Design review of the part built by this model. Coordinates are the model's own, in mm. A direction names the side the tool comes from. Coordinates: 2 decimals unless noted, no trailing zeros. Write each loop counter-clockwise with the first axis right and the second up, starting at its lowest first coordinate (ties: lowest second). Pieces come first, ordered by that corner, then holes. Notation, with made-up numbers: (12, -17.75) -> (31, -17.75) arc R26 cw to (31, 19.25) -> close; hole circle Ø2 at (-20.5, 26.5). An arc over 180 degrees is marked (long way). Answer in a Markdown table with one row per item. Add a question column.
Item 1: Take a section at A-A, the plane x = 0. Give the number of separate pieces and of enclosed holes in the cut face, and give its area (3 significant figures).
Item 2: To check wall thickness, follow line 1 (Z direction, x = -0.05, y = 2.05); line 2 (X direction, y = 3.2, z = 0) (3 decimals); line 3 (Z direction, x = -0.1, y = 0.2). State the ranges of each line that lie inside material, in increasing order.
Item 3: Take a section at B-B, the plane z = 0. Write out the cut boundary in (x, y) (3 decimals), and give its area (4 significant figures).
Item 4: Clearance check with flat-ended pins moving along their axes: P1, Ø1.6, axis at x = 0, z = 0, coming from the +Y side; P2, Ø2.5, axis at x = 0, z = 0, coming from the +Y side; P3, Ø3.5, axis at x = 0, z = 0, coming from the -Y side; P4, Ø3, axis at x = -0.5, z = -9.5, coming from the -Y side. State where each tip first meets the part, or that it passes through.
Item 5: Take a section at D-D, the plane x = 1.35. Write out the cut boundary in (y, z), and give its area (3 significant figures).
Item 6: Draft analysis for pull direction Z (two halves, no side actions). For faces 1 (the face through (-1.391, 2.114, 2.573)), 2 (the face through (0.135, 2.662, -12.996)), 3 (the face through (-2.45, 2.64, -7)), state which applies: released by +Z, released by -Z, zero draft, split by the parting line, or undercut.
Item 7: For faces 4 (the face through (-2.44, 3.89, -0.54)), 5 (the face through (-1, 0, 2)), list the 3-axis set-ups (+Z, -Z, +X, -X, +Y, -Y) from which the entire face can be reached by the end or side of a thin tool; tool diameter is ignored.
Item 8: Take a section at C-C, the plane y = 3.75. Write out the cut boundary in (x, z), and give its area (3 significant figures).
from build123d import *

# Parameters (mm, degrees)
SKETCH1_R           = 2.925
SKETCH1_R_2         = 1.925
BOSS_EXTRUDE1_DEPTH = 1.8
BOSS_EXTRUDE2_DEPTH = 1.7
SKETCH4_R           = 2.5
SKETCH4_R_2         = 2
BOSS_EXTRUDE3_DEPTH = 0.8
SKETCH5_R           = 0.45
CUT_EXTRUDE1_DEPTH  = 17.133234332
SKETCH6_R           = 0.875
CUT_EXTRUDE2_DEPTH  = 17.133234332
SKETCH7_R           = 1.925
CUT_EXTRUDE3_DEPTH  = 1.1
CUT_EXTRUDE4_START  = -0.5
SKETCH8_R           = 2
CUT_EXTRUDE4_DEPTH  = 0.5


with BuildPart() as part:
    # Sketch1 → Boss-Extrude1 (new body)
    with BuildSketch(Plane(origin=(0, 0, 0), x_dir=(1, 0, 0), z_dir=(0, 1, 0))):
        with Locations(Location((0, 0, 0), (0, 0, 270))):
            Circle(SKETCH1_R)
        with Locations(Location((0, 0, 0), (0, 0, 270))):
            Circle(SKETCH1_R_2, mode=Mode.SUBTRACT)
    extrude(amount=BOSS_EXTRUDE1_DEPTH)

    # Sketch3 → Boss-Extrude2 (add)
    with BuildSketch(Plane(origin=(0, 1.8, 0), x_dir=(1, 0, 0), z_dir=(0, 1, 0))):
        with BuildLine():
            Line((2.918100235, 0.200788497), (1.995282212, 13.61229128))
            ThreePointArc((1.995282212, 13.61229128), (0, 15.475), (-1.995282212, 13.61229128))
            Line((-1.995282212, 13.61229128), (-2.918100235, 0.200788497))
            ThreePointArc((-2.918100235, 0.200788497), (0, -2.925), (2.918100235, 0.200788497))
        make_face()
    extrude(amount=BOSS_EXTRUDE2_DEPTH)

    # Sketch4 → Boss-Extrude3 (add)
    with BuildSketch(Plane(origin=(0, 3.5, 0), x_dir=(1, 0, 0), z_dir=(0, 1, 0))):
        with Locations(Location((0, 0, 0), (0, 0, 270))):
            Circle(SKETCH4_R)
        with Locations(Location((0, 0, 0), (0, 0, 270))):
            Circle(SKETCH4_R_2, mode=Mode.SUBTRACT)
    extrude(amount=BOSS_EXTRUDE3_DEPTH)

    # Sketch5 → Cut-Extrude1 (cut, through all)
    with BuildSketch(Plane(origin=(0, 3.5, 0), x_dir=(1, 0, 0), z_dir=(0, 1, 0))):
        with Locations(Location((0, 13.425, 0), (0, 0, 270))):
            Circle(SKETCH5_R)
        with Locations(Location((0, 10.475, 0), (0, 0, 270))):
            Circle(SKETCH5_R)
        with Locations(Location((0, 7.525, 0), (0, 0, 270))):
            Circle(SKETCH5_R)
    extrude(amount=-CUT_EXTRUDE1_DEPTH, mode=Mode.SUBTRACT)

    # Sketch6 → Cut-Extrude2 (cut, through all)
    with BuildSketch(Plane(origin=(0, 3.5, 0), x_dir=(1, 0, 0), z_dir=(0, 1, 0))):
        with Locations(Location((0, 0, 0), (0, 0, 270))):
            Circle(SKETCH6_R)
    extrude(amount=-CUT_EXTRUDE2_DEPTH, mode=Mode.SUBTRACT)

    # Sketch7 → Cut-Extrude3 (cut)
    with BuildSketch(Plane.XZ.offset(-1.8)):
        with Locations(Location((0, 0, 0), (0, 0, 270))):
            Circle(SKETCH7_R)
    extrude(amount=-CUT_EXTRUDE3_DEPTH, mode=Mode.SUBTRACT)

    # Sketch8 → Cut-Extrude4 (cut)
    with BuildSketch(Plane(origin=(0, 3.5, 0), x_dir=(1, 0, 0), z_dir=(0, 1, 0)).offset(CUT_EXTRUDE4_START)):
        with Locations(Location((0, 0, 0), (0, 0, 270))):
            Circle(SKETCH8_R)
    extrude(amount=CUT_EXTRUDE4_DEPTH, mode=Mode.SUBTRACT)


solid = part.part
Answers:
| question | item | result |
|---|---|---|
| 1 | separate pieces | 5 |
| 1 | enclosed holes | 0 |
| 1 | area | 24.7 mm^2 |
| 2 | line 1 | z = -15.47 to -13.87, -12.98 to -10.92, -10.03 to -7.97, -7.08 to -1.92, 1.92 to 2.92 |
| 2 | line 2 | x = -2.925 to -2, 2 to 2.925 |
| 2 | line 3 | z = -2.92 to -1.92, 1.92 to 2.92 |
| 3 | outline | (-2.925, 0) -> (-1.925, 0) -> (-1.925, 2.9) -> (-0.875, 2.9) -> (-0.875, 3) -> (-2, 3) -> (-2, 4.3) -> (-2.5, 4.3) -> (-2.5, 3.5) -> (-2.925, 3.5) -> close; (0.875, 2.9) -> (1.925, 2.9) -> (1.925, 0) -> (2.925, 0) -> (2.925, 3.5) -> (2.5, 3.5) -> (2.5, 4.3) -> (2, 4.3) -> (2, 3) -> (0.875, 3) -> close |
| 3 | area | 7.935 mm^2 |
| 4 | P1 | passes through |
| 4 | P2 | stops at y = 3 |
| 4 | P3 | stops at y = 2.9 |
| 4 | P4 | stops at y = 1.8 |
| 5 | outline | (0, -2.59) -> (1.8, -2.59) -> (1.8, -14.95) -> (3.5, -14.95) -> (3.5, -2.1) -> (4.3, -2.1) -> (4.3, -1.48) -> (3, -1.48) -> (3, 1.48) -> (4.3, 1.48) -> (4.3, 2.1) -> (3.5, 2.1) -> (3.5, 2.59) -> (0, 2.59) -> (0, 1.37) -> (2.9, 1.37) -> (2.9, -1.37) -> (0, -1.37) -> close |
| 5 | area | 30.7 mm^2 |
| 6 | face 1 | split by the parting line |
| 6 | face 2 | undercut |
| 6 | face 3 | released by -Z |
| 7 | face 4 | +Y |
| 7 | face 5 | +Z, -Z, +X, -X, -Y |
| 8 | outline | circle Ø5 at (0, 0); hole circle Ø4 at (0, 0) |
| 8 | area | 7.07 mm^2 |
